Part model, mm, in its own coordinate system. A direction names the side the tool comes from. Give positions to 0.01 mm unless a question says otherwise; leave off trailing zeros. Write each loop counter-clockwise with the first axis right and the second up, starting at its lowest first coordinate (ties: lowest second). Pieces come first, ordered by that corner, then holes. Notation, with made-up numbers: (-14, -15.75) - (0, -15.75) arc R6 ccw to (0, -8.75) - close; hole circle Ø6 at (63, -19). An arc over 180 degrees is marked (long way). Answer as a JSON object with one key per item and string values. Group by question number.
```python
from build123d import *

# Parameters (mm, degrees)
SKETCH1_W           = 40
SKETCH1_H           = 30
SKETCH1_W_2         = 30
SKETCH1_H_2         = 20
BOSS_EXTRUDE1_DEPTH = 20
SKETCH2_W           = 10
SKETCH2_H           = 10
SKETCH2_R           = 1.25
BOSS_EXTRUDE2_DEPTH = 4
FILLET1_START       = 16
FILLET1_DEPTH       = 4
FILLET1_2_DEPTH     = 4
SKETCH3_W           = 40
SKETCH3_H           = 20
SKETCH3_W_2         = 30
SKETCH3_H_2         = 10.847900724
BOSS_EXTRUDE3_DEPTH = 5
SKETCH4_W           = 15
SKETCH4_H           = 5
BOSS_EXTRUDE4_DEPTH = 5


with BuildPart() as part:
    # Sketch1 → Boss-Extrude1 (new body)
    with BuildSketch(Plane.XY):
        Rectangle(SKETCH1_W, SKETCH1_H)
        Rectangle(SKETCH1_W_2, SKETCH1_H_2, mode=Mode.SUBTRACT)
    extrude(amount=BOSS_EXTRUDE1_DEPTH)

    # Sketch2 → Boss-Extrude2 (add)
    # profile 1 of 2: a face of its own
    with BuildSketch(Plane.XY.offset(20)):
        with Locations((-25, 0)):
            Rectangle(SKETCH2_W, SKETCH2_H)
        with Locations((-25, 0)):
            Circle(SKETCH2_R, mode=Mode.SUBTRACT)
    # profile 2 of 2: a face of its own
    with BuildSketch(Plane.XY.offset(20)):
        with Locations((25, 0)):
            Rectangle(SKETCH2_W, SKETCH2_H)
        with Locations(Location((25, 0, 0), (0, 0, 180))):
            Circle(SKETCH2_R, mode=Mode.SUBTRACT)
    extrude(amount=-BOSS_EXTRUDE2_DEPTH)

    # Fillet1: read off the stored shape, not the designer's step
    # Fillet1 outline → Fillet1 (cut)
    with BuildSketch(Plane.XY.offset(FILLET1_START)):
        with BuildLine():
            ThreePointArc((30, 0), (28.535533906, -3.535533906), (25, -5))
            Line((25, -5), (30, -5))
            Line((30, -5), (30, 0))
        make_face()
        with BuildLine():
            ThreePointArc((25, 5), (28.535533906, 3.535533906), (30, 0))
            Line((30, 0), (30, 5))
            Line((30, 5), (25, 5))
        make_face()
        with BuildLine():
            ThreePointArc((-30, 0), (-28.535533906, 3.535533906), (-25, 5))
            Line((-25, 5), (-30, 5))
            Line((-30, 5), (-30, 0))
        make_face()
        with BuildLine():
            ThreePointArc((-25, -5), (-28.535533906, -3.535533906), (-30, 0))
            Line((-30, 0), (-30, -5))
            Line((-30, -5), (-25, -5))
        make_face()
    extrude(amount=FILLET1_DEPTH, mode=Mode.SUBTRACT)

    # Fillet1 2 outline → Fillet1 2 (add)
    with BuildSketch(Plane.XY.offset(FILLET1_START)):
        with BuildLine():
            ThreePointArc((20, -10), (21.464466094, -6.464466094), (25, -5))
            Line((25, -5), (20, -5))
            Line((20, -5), (20, -10))
        make_face()
        with BuildLine():
            Line((20, 5), (25, 5))
            ThreePointArc((25, 5), (21.464466094, 6.464466094), (20, 10))
            Line((20, 10), (20, 5))
        make_face()
        with BuildLine():
            ThreePointArc((-20, 10), (-21.464466094, 6.464466094), (-25, 5))
            Line((-25, 5), (-20, 5))
            Line((-20, 5), (-20, 10))
        make_face()
        with BuildLine():
            Line((-20, -5), (-25, -5))
            ThreePointArc((-25, -5), (-21.464466094, -6.464466094), (-20, -10))
            Line((-20, -10), (-20, -5))
        make_face()
    extrude(amount=FILLET1_2_DEPTH)

    # Sketch3 → Boss-Extrude3 (add)
    with BuildSketch(Plane.XZ.offset(15)):
        with Locations((0, -10)):
            Rectangle(SKETCH3_W, SKETCH3_H)
        with Locations((0, -9.576049638)):
            Rectangle(SKETCH3_W_2, SKETCH3_H_2, mode=Mode.SUBTRACT)
    extrude(amount=-BOSS_EXTRUDE3_DEPTH)

    # Sketch4 → Boss-Extrude4 (add)
    with BuildSketch(Plane(origin=(0, 0, -20), x_dir=(-1, 0, 0), z_dir=(0, 0, -1))):
        Polygon((20, 40), (15, 40), (15, 35), (15, -10), (20, -10), align=None)
        with Locations((7.5, 37.5)):
            Rectangle(SKETCH4_W, SKETCH4_H)
        with Locations((-7.5, 37.5)):
            Rectangle(SKETCH4_W, SKETCH4_H)
        Polygon((-15, 35), (-15, 40), (-20, 40), (-20, -10), (-15, -10), align=None)
    extrude(amount=-BOSS_EXTRUDE4_DEPTH)


solid = part.part
```
1) Drop flat-ended pins along their axis: P1, Ø2, axis at x = -10, z = -2, coming from the +Y side; P2, Ø5.5, axis at y = 3.5, z = -18.5, coming from the -X side; P3, Ø5, axis at x = 26.5, y = -4.5, coming from the -Z side; P4, Ø1, axis at x = -9, y = 16, coming from the -Z side. Give the stop position or say it passes through.
2) Saw through at B-B (x = 12.5). List the corners of the cut face in (y, z).
3) Which spindle directions (+Z, -Z, +X, -X, +Y, -Y) get a long thin tool onto all of the face, cutting with end or side? Do faces 5 (the flat face through (23, 0, 16)), 6 (the flat face through (-15, 0, 10)), 7 (the flat face through (0, 11, 0)), 8 (the flat face through (0, -13, -4.152)). Say none if no direction does.
4) Two-plate mould, pull along Y, no slides. Class faces 1 (the flat face through (0, 15, 10)), 2 (the flat face through (0, -10, -17)), 3 (the flat face through (0, -15, 5)), 4 (the flat face through (18, 13, -20)): +Y half, -Y half, draft (parallel to the pull), parting line (faces both ways), or undercut.
5) Saw through at D-D (z = 14.5). List the corners of the cut face in (x, y), and give its area (3 significant figures).
6) Saw through at C-C (z = -6.5). List the corners of the cut face in (x, y), and give its area (3 significant figures).
7) Saw through at A-A (y = 19). List the corners of the cut face in (x, z).
8) Drill centre lines: line 1 along Z through (x, y) = (19.5, -7); line 2 along Y through (x, z) = (-25, 18.85); line 3 along X through (y, z) = (6.5, 11). Where is each one in solid material? Low to high. Write a range as from..to.
Checks:
{
 "1": {"P1": "y = -10", "P2": "x = -20", "P3": "z = 16", "P4": "through"},
 "2": {"outline": "(-15, -20) - (-10, -20) - (-10, -15) - (-15, -15) - close; (-15, -4.15) - (-10, -4.15) - (-10, 20) - (-15, 20) - close; (10, 0) - (15, 0) - (15, 20) - (10, 20) - close; (35, -20) - (40, -20) - (40, -15) - (35, -15) - close"},
 "3": {"face 5": "-Z, +X, +Y, -Y", "face 6": "+Z, -Z", "face 7": "+X, -X, +Y", "face 8": "+Y, -Y"},
 "4": {"face 1": "+Y half", "face 2": "undercut", "face 3": "-Y half", "face 4": "draft"},
 "5": {"outline": "(-20, -15) - (20, -15) - (20, 15) - (-20, 15) - close; hole (-15, -10) - (15, -10) - (15, 10) - (-15, 10) - close", "area": "600 mm2"},
 "6": {"outline": "(-20, -15) - (-15, -15) - (-15, -10) - (-20, -10) - close; (15, -15) - (20, -15) - (20, -10) - (15, -10) - close", "area": "50.0 mm2"},
 "7": {"outline": "(-20, -20) - (-15, -20) - (-15, -15) - (-20, -15) - close; (15, -20) - (20, -20) - (20, -15) - (15, -15) - close"},
 "8": {"line 1": "-20..-15, 0..20", "line 2": "-5..-1.25, 1.25..5", "line 3": "-20..-15, 15..20"}
}
